Model file for the job. Use its own axes, mm. A direction names the side the tool comes from. Coordinates: 2 decimals unless noted, no trailing zeros. Write each loop counter-clockwise with the first axis right and the second up, starting at its lowest first coordinate (ties: lowest second). Pieces come first, ordered by that corner, then holes. Notation, with made-up numbers: M 18,34 L 25,34 A19 cw 25,64 Z; hole C 74.25,17 d5. An arc over 180 degrees is marked long. Put each result on its own line as item: value. Start each with the question number.
Q1. Drill centre lines: line 1 along Y through (x, z) = (22, 1.6); line 2 along X through (y, z) = (-8, 1.25); line 3 along X through (y, z) = (-14, 0.5). Where is each one in solid material? Low to high.
Q2. Drop flat-ended pins along their axis: pin 1 (1 mm diameter, centred on x = -14, y = 14, fed in from -Z); pin 2 (0.9 mm diameter, centred on x = 22.5, z = 1.5, fed in from +Y); pin 3 (1 mm diameter, centred on x = 2.5, z = 1, fed in from -Y); pin 4 (3.5 mm diameter, centred on x = 6, y = -6, fed in from +Z). Give the stop position or say it passes through.
Q3. Cut at A-A (y = -9). Write the cut outline in (x, z).
Q4. Pull direction X, two halves, no side cores. Call faces 4 (the flat face through (-27.5, 0, 1)), 5 (the flat face through (-12, 19, 1)), 6 (the flat face through (26, 18, 2)): pulls with the +X half, pulls with the -X half, needs draft (parallel to the pull), parting line crosses it, or undercut.
Q5. Cut at D-D (y = 13.75). Write the cut outline in (x, z), then the cut area to 3 significant figures.
Q6. Which spindle directions (+Z, -Z, +X, -X, +Y, -Y) get a long thin tool onto all of the face, cutting with end or side? Do faces 1 (the flat face through (0, 0, 2)), 2 (the flat face through (-26, -18, 2)), 3 (the flat face through (26.5, 8, 2)). Say none if no direction does.
Q7. Cut at B-B (x = 16). Write the cut outline in (y, z).
Q8. Cut at C-C (z = 1.45). Give the number of separate pieces and of enclosed holes in the cut face, then the cut area to 3 significant figures.
```python
from build123d import *

# Parameters (mm, degrees)
SKETCH_1_W          = 55
SKETCH_1_H          = 38
EXTRUDE_1_DEPTH     = 3
SKETCH_2_R          = 1.5
CUT_EXTRUDE_1_DEPTH = 30
SKETCH_3_W          = 8
SKETCH_3_H          = 3
CUT_EXTRUDE_2_DEPTH = 30
SKETCH_4_W          = 20
SKETCH_4_H          = 38
CUT_EXTRUDE_3_DEPTH = 1
SKETCH_5_W          = 9
SKETCH_5_H          = 4
CUT_EXTRUDE_4_DEPTH = 10
SKETCH_6_W          = 12
SKETCH_6_H          = 3
CUT_EXTRUDE_5_DEPTH = 10
SKETCH_8_R          = 1.5
CUT_EXTRUDE_6_DEPTH = 10
SKETCH_9_R          = 0.5
CUT_EXTRUDE_7_DEPTH = 4


with BuildPart() as part:
    # 草图1 → 凸台-拉伸1 (new body)
    with BuildSketch(Plane.XY):
        Rectangle(SKETCH_1_W, SKETCH_1_H)
    extrude(amount=EXTRUDE_1_DEPTH)

    # 草图2 → 切除-拉伸1 (cut)
    with BuildSketch(Plane.XY.offset(3)):
        with Locations((16, 13.75)):
            Circle(SKETCH_2_R)
        with Locations((16, -13.75)):
            Circle(SKETCH_2_R)
        with Locations((-16, 13.75)):
            Circle(SKETCH_2_R)
        with Locations((-16, -13.75)):
            Circle(SKETCH_2_R)
    extrude(amount=-CUT_EXTRUDE_1_DEPTH, mode=Mode.SUBTRACT)

    # 草图3 → 切除-拉伸2 (cut)
    with BuildSketch(Plane.XY.offset(3)):
        with Locations((22, 17.5)):
            Rectangle(SKETCH_3_W, SKETCH_3_H)
        with Locations((22, -17.5)):
            Rectangle(SKETCH_3_W, SKETCH_3_H)
        with Locations((-22, 17.5)):
            Rectangle(SKETCH_3_W, SKETCH_3_H)
        with Locations((-22, -17.5)):
            Rectangle(SKETCH_3_W, SKETCH_3_H)
    extrude(amount=-CUT_EXTRUDE_2_DEPTH, mode=Mode.SUBTRACT)

    # 草图4 → 切除-拉伸3 (cut)
    with BuildSketch(Plane.XY.offset(3)):
        Rectangle(SKETCH_4_W, SKETCH_4_H)
    extrude(amount=-CUT_EXTRUDE_3_DEPTH, mode=Mode.SUBTRACT)

    # 草图5 → 切除-拉伸4 (cut)
    with BuildSketch(Plane.XY.offset(3)):
        with Locations((22, 8)):
            Rectangle(SKETCH_5_W, SKETCH_5_H)
        with Locations((22, 0)):
            Rectangle(SKETCH_5_W, SKETCH_5_H)
        with Locations((22, -8)):
            Rectangle(SKETCH_5_W, SKETCH_5_H)
        with Locations((-22, -8)):
            Rectangle(SKETCH_5_W, SKETCH_5_H)
        with Locations((-22, 8)):
            Rectangle(SKETCH_5_W, SKETCH_5_H)
        with Locations((-22, 0)):
            Rectangle(SKETCH_5_W, SKETCH_5_H)
    extrude(amount=-CUT_EXTRUDE_4_DEPTH, mode=Mode.SUBTRACT)

    # 草图6 → 切除-拉伸5 (cut)
    with BuildSketch(Plane.XY.offset(2)):
        with Locations((0, 17.5)):
            Rectangle(SKETCH_6_W, SKETCH_6_H)
        with Locations((0, -17.5)):
            Rectangle(SKETCH_6_W, SKETCH_6_H)
    extrude(amount=-CUT_EXTRUDE_5_DEPTH, mode=Mode.SUBTRACT)

    # 草图8 → 切除-拉伸6 (cut)
    with BuildSketch(Plane.XY.offset(2)):
        with Locations((6, -6)):
            Circle(SKETCH_8_R)
        with Locations((6, 6)):
            Circle(SKETCH_8_R)
        with Locations((-6, 6)):
            Circle(SKETCH_8_R)
        with Locations((-6, -6)):
            Circle(SKETCH_8_R)
    extrude(amount=-CUT_EXTRUDE_6_DEPTH, mode=Mode.SUBTRACT)

    # 草图9 → 切除-拉伸7 (cut, through all)
    with BuildSketch(Plane.XY.offset(3)):
        with Locations((25.787867966, -16.212132034)):
            Circle(SKETCH_9_R)
        with Locations((18.212132034, -16.212132034)):
            Circle(SKETCH_9_R)
        with Locations((18.212132034, 16.212132034)):
            Circle(SKETCH_9_R)
        with Locations((25.787867966, 16.212132034)):
            Circle(SKETCH_9_R)
        with Locations((-25.787867966, 16.212132034)):
            Circle(SKETCH_9_R)
        with Locations((-18.212132034, 16.212132034)):
            Circle(SKETCH_9_R)
        with Locations((-18.212132034, -16.212132034)):
            Circle(SKETCH_9_R)
        with Locations((-25.787867966, -16.212132034)):
            Circle(SKETCH_9_R)
        with Locations((5.787867966, -16.212132034)):
            Circle(SKETCH_9_R)
        with Locations((-5.787867966, -16.212132034)):
            Circle(SKETCH_9_R)
        with Locations((-5.787867966, 16.212132034)):
            Circle(SKETCH_9_R)
        with Locations((5.787867966, 16.212132034)):
            Circle(SKETCH_9_R)
    extrude(amount=-CUT_EXTRUDE_7_DEPTH, mode=Mode.SUBTRACT)


solid = part.part
```
Computed values:
1. line 1: -16 to -10, -6 to -2, 2 to 6, 10 to 16
1. line 2: -27.5 to -26.5, -17.5 to 17.5, 26.5 to 27.5
1. line 3: -27.5 to -17.48, -14.52 to 14.52, 17.48 to 27.5
2. pin 1: z = 0
2. pin 2: y = 16
2. pin 3: y = -16
2. pin 4: z = 2
3. outline: M -27.5,0 L -26.5,0 L -26.5,3 L -27.5,3 Z; M -17.5,0 L 17.5,0 L 17.5,3 L 10,3 L 10,2 L -10,2 L -10,3 L -17.5,3 Z; M 26.5,0 L 27.5,0 L 27.5,3 L 26.5,3 Z
4. face 4: pulls with the -X half
4. face 5: needs draft
4. face 6: undercut
5. outline: M -27.5,0 L -17.5,0 L -17.5,3 L -27.5,3 Z; M -14.5,0 L 14.5,0 L 14.5,3 L 10,3 L 10,2 L -10,2 L -10,3 L -14.5,3 Z; M 17.5,0 L 27.5,0 L 27.5,3 L 17.5,3 Z
5. area: 127 mm2
6. face 1: +Z, +Y, -Y
6. face 2: +Z, -Z, -Y
6. face 3: +Z, -Z
7. outline: M -19,0 L -15.25,0 L -15.25,3 L -19,3 Z; M -12.25,0 L 12.25,0 L 12.25,3 L -12.25,3 Z; M 15.25,0 L 19,0 L 19,3 L 15.25,3 Z
8. separate pieces: 1
8. enclosed holes: 14
8. area: 1,650 mm2
